Could you check a few things on this model? Use its own coordinates, in mm. A direction names the side the tool comes from. Round coordinates to 2 decimals unless told otherwise and drop trailing zeros. Loops run counter-clockwise (first coordinate to the right, second up) from the corner with the lowest first, then second, coordinate; pieces in that order, holes last. Notation, with made-up numbers: M 28,-7 L 81,-7 A31 ccw 81,20 Z; hole C 19.5,25 d1. An arc over 180 degrees is marked long. One line per item, written item: value. Start each with the question number.
Q1. Imagine slicing it at C-C (x = -6.25). Please give me the cut outline in (y, z) (3 decimals).
Q2. Please list where these lines run through material, in increasing order: line 1 along X through (y, z) = (-0.75, -1.5) (3 decimals); line 2 along Y through (x, z) = (-2.7, 0.5); line 3 along Z through (x, y) = (-8.5, -1.75).
Q3. Imagine slicing it at B-B (y = -0.5). Please give me the cut outline in (x, z).
Q4. Imagine slicing it at A-A (z = -1.25). Please give me the cut outline in (x, y).
Q5. Which directions (+Z, -Z, +X, -X, +Y, -Y) give clear straight access to the entire face, cutting with the end or side of a thin tool? Please do faces 4 (the face through (3.52, -0.64, 0.64)), 5 (the face through (-2, 0, 3.95)), 6 (the face through (-2.6, 1, -3.6)), 7 (the face through (-0.981, -3.414, -0.055)).
Q6. Imagine slicing it at D-D (x = 2). Please give me the cut outline in (y, z), then the cut area to 3 significant figures.
Q7. I'm going to push flat-ended pins straight in: pin 1 Ø0.9 at (x, z) = (-7, 0) entering from +Y; pin 2 Ø4.5 at (x, y) = (2.5, 1) entering from -Z; pin 3 Ø2 at (y, z) = (-3.5, -0.5) entering from -X; pin 4 Ø1.8 at (x, y) = (-2.7, -1.7) entering from +Z. Where does each tip first touch, or does it pass through?
Q8. Thinking about a two-plate mould opening in Y: for faces 1 (the face through (-12.1, 3.12, 0.04)), 2 (the face through (0, -2, 1)), 3 (the face through (-10.968, 0.779, 2.947)), which applies, released by +Y, released by -Y, zero draft, split by the parting line, or undercut?
from build123d import *

# Parameters (mm, degrees)
BOSS_EXTRUDE1_DEPTH     = 3.2
BOSS_EXTRUDE2_DEPTH     = 0.75
CUT_EXTRUDE1_DEPTH      = 16.439388307
CUT_EXTRUDE1_DEPTH_BACK = 16.439388307
SKETCH4_R               = 1.5
BOSS_EXTRUDE3_DEPTH     = 6.3
CHAMFER1_SIZE           = 0.5
CHAMFER2_SIZE           = 0.5
CUT_EXTRUDE2_DEPTH      = 5.2


with BuildPart() as part:
    # Sketch1 → Boss-Extrude1 (new, symmetric)
    with BuildSketch(Plane.XY):
        Polygon((-10, -4.4), (10, -4.4), (10, -1.4), (0, 2.6), (-10, 4.4), (-10, -0.2), align=None)
        Polygon((-12.394804782, 1.478031011), (-10, -0.2), (-10, 4.4), (-11.810199888, 4.72583598), align=None)
    extrude(amount=BOSS_EXTRUDE1_DEPTH, both=True)

    # Sketch2 → Boss-Extrude2 (add, symmetric)
    with BuildSketch(Plane.XY.offset(3.2)):
        with BuildLine():
            ThreePointArc((0, -1.7), (-2.7, 1), (-5.4, -1.7))
            Line((-5.4, -1.7), (-2.7, -4.4))
            Line((-2.7, -4.4), (0, -1.7))
        make_face()
        with BuildLine():
            Line((-2.7, -4.4), (-5.4, -1.7))
            ThreePointArc((-5.4, -1.7), (-4.609188309, -3.609188309), (-2.7, -4.4))
        make_face()
        with BuildLine():
            Line((0, -1.7), (-2.7, -4.4))
            ThreePointArc((-2.7, -4.4), (-0.790811691, -3.609188309), (0, -1.7))
        make_face()
        with BuildLine():
            ThreePointArc((0, -1.7), (-0.790811691, -3.609188309), (-2.7, -4.4))
            Line((-2.7, -4.4), (0, -4.4))
            Line((0, -4.4), (0, -1.7))
        make_face()
        with BuildLine():
            ThreePointArc((-2.7, -4.4), (-4.609188309, -3.609188309), (-5.4, -1.7))
            Line((-5.4, -1.7), (-5.4, -4.4))
            Line((-5.4, -4.4), (-2.7, -4.4))
        make_face()
    boss_extrude2 = extrude(amount=BOSS_EXTRUDE2_DEPTH, both=True)

    # Mirror1: Boss-Extrude2 across plane
    add(boss_extrude2.mirror(Plane.XY))

    # Sketch3 → Cut-Extrude1 (cut, two sides: drawn at the far end of the back side and taken through both)
    with BuildSketch(Plane.XY.offset(3.95).offset(-CUT_EXTRUDE1_DEPTH_BACK)):
        with BuildLine():
            ThreePointArc((-1.2, -1.7), (-3.060572549, -0.243982336), (-4.026649916, -2.4))
            Line((-4.026649916, -2.4), (-1.373350084, -2.4))
            ThreePointArc((-1.373350084, -2.4), (-1.243982336, -2.060572549), (-1.2, -1.7))
        make_face()
        with BuildLine():
            Line((-1.373350084, -2.4), (-4.026649916, -2.4))
            ThreePointArc((-4.026649916, -2.4), (-2.7, -3.2), (-1.373350084, -2.4))
        make_face()
        with BuildLine():
            Line((-4.026649916, -2.4), (-4.8, -4.4))
            Line((-4.8, -4.4), (-0.6, -4.4))
            Line((-0.6, -4.4), (-1.373350084, -2.4))
            ThreePointArc((-1.373350084, -2.4), (-2.7, -3.2), (-4.026649916, -2.4))
        make_face()
    extrude(amount=CUT_EXTRUDE1_DEPTH + CUT_EXTRUDE1_DEPTH_BACK, mode=Mode.SUBTRACT)

    # Sketch4 → Boss-Extrude3 (add, symmetric)
    with BuildSketch(Plane.XY):
        with Locations((10, -2.9)):
            Circle(SKETCH4_R)
    extrude(amount=BOSS_EXTRUDE3_DEPTH, both=True)

    # Chamfer1
    chamfer1_edges = [part.edges().sort_by_distance(p)[0] for p in [
        (8.5, -2.9, -6.3),
        (8.5, -2.9, 6.3),
    ]]
    chamfer(chamfer1_edges, length=CHAMFER1_SIZE)

    # Chamfer2
    chamfer2_edges = [part.edges().sort_by_distance(p)[0] for p in [
        (-5.905099944, 3.66291799, 3.2),
        (-11.197402391, 0.639015505, -3.2),
        (-12.102502335, 3.101933495, -3.2),
        (-5.905099944, 3.66291799, -3.2),
        (5, 0.6, -3.2),
        (-12.102502335, 3.101933495, 3.2),
        (-11.197402391, 0.639015505, 3.2),
        (-10, -2.3, 3.2),
        (5, 0.6, 3.2),
        (-10, -2.3, -3.2),
    ]]
    chamfer(chamfer2_edges, length=CHAMFER2_SIZE)

    # Sketch5 → Cut-Extrude2 (cut)
    with BuildSketch(Plane.XY.offset(3.2)):
        with BuildLine():
            Line((-10.438248334, 2.751564232), (-10.529148071, 2.246565691))
            Line((-10.529148071, 2.246565691), (-8.3, 0.684609736))
            Line((-8.3, 0.684609736), (-8.3, -3.2))
            Line((-8.3, -3.2), (-5.4, -3.2))
            Line((-5.4, -3.2), (-5.4, -1.7))
            ThreePointArc((-5.4, -1.7), (-2.7, 1), (0, -1.7))
            Line((0, -1.7), (0, -3.2))
            Line((0, -3.2), (7.316718427, -3.2))
            ThreePointArc((7.316718427, -3.2), (7.308115775, -2.690812714), (7.395278362, -2.189067379))
            Line((7.395278362, -2.189067379), (-0.471070755, 0.957472268))
            Line((-0.471070755, 0.957472268), (-10.438248334, 2.751564232))
        make_face()
    extrude(amount=-CUT_EXTRUDE2_DEPTH, mode=Mode.SUBTRACT)


solid = part.part
Report:
1. outline: M -4.4,-3.2 L 3.217,-3.2 L 3.725,-2.7 L 3.725,2.7 L 3.217,3.2 L 1.998,3.2 L 1.998,-2 L -3.2,-2 L -3.2,3.2 L -4.4,3.2 Z
2. line 1: x = -10 to -8.3, -5.227 to -3.861, -1.539 to -0.173, 3.798 to 8.375
2. line 2: y = -0.2 to 1, 1.36 to 3.09
2. line 3: z = -3.2 to 3.2
3. outline: M -10,-2.7 L -9.5,-3.2 L -5.12,-3.2 L -5.12,-3.95 L -3.6,-3.95 L -3.6,3.95 L -5.12,3.95 L -5.12,-2 L -8.3,-2 L -8.3,3.2 L -9.5,3.2 L -10,2.7 Z; M -1.8,-3.95 L -0.28,-3.95 L -0.28,-3.2 L 6.4,-3.2 L 7.75,-2.7 L 7.75,2.7 L 6.4,3.2 L 3.17,3.2 L 3.17,-2 L -0.28,-2 L -0.28,3.95 L -1.8,3.95 Z
4. outline: M -12.39,1.48 L -10,-0.2 L -10,-4.4 L -4.8,-4.4 L -4.03,-2.4 A1.5 cw long -1.37,-2.4 L -0.6,-4.4 L 10,-4.4 A1.5 ccw 10,-1.4 L 0,2.6 L -11.81,4.73 Z; hole M -10.53,2.25 L -8.3,0.68 L -8.3,-3.2 L -5.4,-3.2 L -5.4,-1.7 A2.7 cw 0,-1.7 L 0,-3.2 L 7.32,-3.2 A2.7 cw 7.4,-2.19 L -0.47,0.96 L -10.44,2.75 Z
5. face 4: +Z
5. face 5: +Z, -X, +Y, -Y
5. face 6: -Z, +Y
5. face 7: +Z, -Z, -Y
6. outline: M -4.4,-3.2 L 1.26,-3.2 L 1.8,-2.7 L 1.8,2.7 L 1.26,3.2 L -0.03,3.2 L -0.03,-2 L -3.2,-2 L -3.2,3.2 L -4.4,3.2 Z
6. area: 22.9 mm²
7. pin 1: stops at y = 3.94
7. pin 2: stops at z = -3.2
7. pin 3: stops at x = -10
7. pin 4: passes through
8. face 1: released by +Y
8. face 2: undercut
8. face 3: released by -Y
